Autodesk Inventor part; units mm, degrees
ref_plane "YZ Plane" through (0, 0, 0) normal (1, 0, 0) x (0, 1, 0)
ref_plane "XZ Plane" through (0, 0, 0) normal (0, 1, 0) x (-1, 0, 0)
ref_plane "XY Plane" through (0, 0, 0) normal (0, 0, 1) x (1, 0, 0)
sketch "Sketch1" plane through (0, 0, 0) normal (0, 0, 1) x (1, 0, 0)
  line L0 (-21.25, 19.05) -> (21.25, 19.05)
  line L1 (21.25, 19.05) -> (21.25, -19.05)
  line L2 (21.25, -19.05) -> (-21.25, -19.05)
  line L3 (-21.25, -19.05) -> (-21.25, 19.05)
  line L4 (21.25, 0) -> (-21.25, 0) construction
  circle A0 centre (19, 0) radius 0.875
  line L5 (-19.445, 0.915) -> (-18.555, 0.915)
  line L6 (-18.555, -0.915) -> (-19.445, -0.915)
  arc A1 (-19.445, 0.915) -> (-19.445, -0.915) centre (-19.445, 0) ccw
  arc A2 (-18.555, -0.915) -> (-18.555, 0.915) centre (-18.555, 0) ccw
  line L7 (0, -19.05) -> (0, 19.05) construction
  line L8 (-19, 0.915) -> (-19, -0.915) construction
  point P0 (0, 0)
  point P1 (-19, 0)
  dimension "d0" = 38.1
  dimension "d2" = 42.5
  dimension "d3" = 2.25
  dimension "d4" = 1.75
  dimension "d6" = 1.83
  dimension "d7" = 2.72
  dimension "d8" = 38
extrude "Extrusion1" add sketch "Sketch1" along normal blind 4.04
sketch "Sketch2" plane through (0, 0, 4.04) normal (0, 0, 1) x (1, 0, 0)
  line L0 (-16.61, 16.61) -> (16.61, 16.61)
  line L1 (16.61, 16.61) -> (16.61, -16.61)
  line L2 (16.61, -16.61) -> (-16.61, -16.61)
  line L3 (-16.61, -16.61) -> (-16.61, 16.61)
  line L4 (0, 16.61) -> (0, -16.61) construction
  line L5 (-16.61, 0) -> (16.61, 0) construction
  point P0 (0, 0)
  dimension "d11" = 33.22
  dimension "d18" = 33.22
extrude "Extrusion2" add sketch "Sketch2" along normal blind 0.61
sketch "Sketch3" plane through (0, 0, 4.65) normal (0, 0, 1) x (1, 0, 0)
  line L0 (16.61, 16.61) -> (-16.61, 16.61)
  line L1 (-16.61, 16.61) -> (-16.61, -16.61)
  line L2 (-16.61, -16.61) -> (16.61, -16.61)
  line L3 (16.61, -16.61) -> (16.61, 16.61)
  line L4 (-9.5505, 7.125) -> (9.5505, 7.125)
  line L5 (9.5505, 7.125) -> (9.5505, -7.125)
  line L6 (9.5505, -7.125) -> (-9.5505, -7.125)
  line L7 (-9.5505, -7.125) -> (-9.5505, 7.125)
  line L8 (-9.5505, 7.125) -> (9.5505, -7.125) construction
  line L9 (9.5505, 7.125) -> (-9.5505, -7.125) construction
  point P0 (0, 0)
  point P1 (0, 0)
  dimension "d21" = 19.101
  dimension "d23" = 14.25
properties part number "KAC12040"
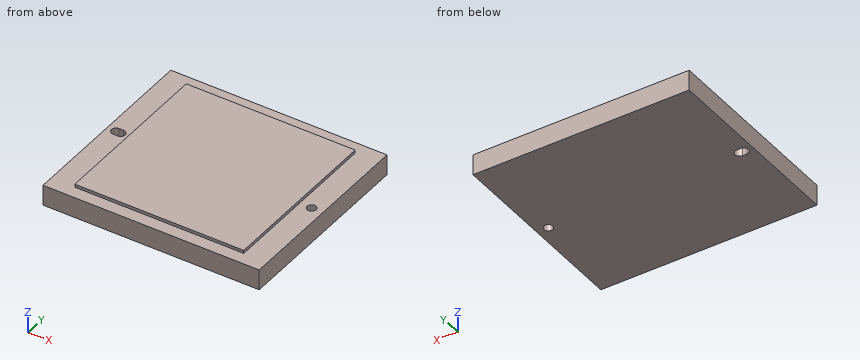
Read the model definition and answer for the solid it produces. Units are mm, in the model's axes. Round coordinates to 2 decimals unless told otherwise and drop trailing zeros. Write each loop counter-clockwise with the first axis right and the second up, starting at its lowest first coordinate (ties: lowest second). Pieces come first, ordered by that corner, then holes.
1. Given pin 1 Ø0.5 at (y, z) = (6.5, 4.5) entering from +X, flat-ended and moving along its own axis, determine where the tip first touches the part or whether it passes through.
2. The part is cut by section D-D, the plane x = -15. Determine the outline of the cut face in (y, z), then the cut area to 3 significant figures.
3. The part is cut by section C-C, the plane y = 6.5. Determine the outline of the cut face in (x, z), then the cut area to 3 significant figures.
4. Straight lines are drawn through the part: L1, parallel to Y at x = 19, z = 1.15 (3 decimals); L2, parallel to Z at x = 17.5, y = 13.5. For each, find the intervals that lie inside material, in ascending order.
5. The part is cut by section A-A, the plane y = 0. Determine the outline of the cut face in (x, z) (3 decimals).
6. The part is cut by section B-B, the plane x = 19. Determine the outline of the cut face in (y, z) (3 decimals), then the cut area to 3 significant figures.
Values:
1. pin 1: stops at x = 16.61
2. outline: (-19.05, 0) - (19.05, 0) - (19.05, 4.04) - (16.61, 4.04) - (16.61, 4.65) - (-16.61, 4.65) - (-16.61, 4.04) - (-19.05, 4.04) - close
2. area: 174 mm2
3. outline: (-21.25, 0) - (21.25, 0) - (21.25, 4.04) - (16.61, 4.04) - (16.61, 4.65) - (-16.61, 4.65) - (-16.61, 4.04) - (-21.25, 4.04) - close
3. area: 192 mm2
4. L1: y = -19.05 to -0.875, 0.875 to 19.05
4. L2: z = 0 to 4.04
5. outline: (-21.25, 0) - (-20.36, 0) - (-20.36, 4.04) - (-21.25, 4.04) - close; (-17.64, 0) - (18.125, 0) - (18.125, 4.04) - (16.61, 4.04) - (16.61, 4.65) - (-16.61, 4.65) - (-16.61, 4.04) - (-17.64, 4.04) - close; (19.875, 0) - (21.25, 0) - (21.25, 4.04) - (19.875, 4.04) - close
6. outline: (-19.05, 0) - (-0.875, 0) - (-0.875, 4.04) - (-19.05, 4.04) - close; (0.875, 0) - (19.05, 0) - (19.05, 4.04) - (0.875, 4.04) - close
6. area: 147 mm2
